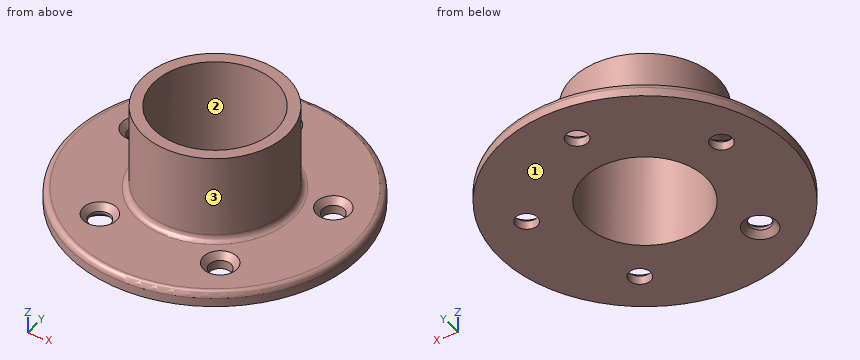
from build123d import *

# Parameters (mm, degrees)
F0_R     = 63.5
F0_R_2   = 4.7625
F0_R_3   = 26.67
F1_DEPTH = 6.35
F2_R     = 31.75
F2_R_2   = 26.67
F3_DEPTH = 38.1
F4_R     = 2.54
F5_SIZE  = 2.54


with BuildPart() as f1:
    # F0 (on Top) → F1 (new body)
    with BuildSketch(Plane.XY):
        Circle(F0_R)
        with Locations((-26.654833, -36.68723)):
            Circle(F0_R_2, mode=Mode.SUBTRACT)
        with Locations((26.654833, -36.68723)):
            Circle(F0_R_2, mode=Mode.SUBTRACT)
        with Locations((-43.128426, 14.013275)):
            Circle(F0_R_2, mode=Mode.SUBTRACT)
        Circle(F0_R_3, mode=Mode.SUBTRACT)
        with Locations((43.128426, 14.013275)):
            Circle(F0_R_2, mode=Mode.SUBTRACT)
        with Locations((0, 45.34791)):
            Circle(F0_R_2, mode=Mode.SUBTRACT)
    extrude(amount=F1_DEPTH)

    # F2 (on face) → F3 (join)
    with BuildSketch(Plane.XY.offset(6.35)):
        Circle(F2_R)
        Circle(F2_R_2, mode=Mode.SUBTRACT)
    extrude(amount=F3_DEPTH)

    # F4
    f4_edges = [f1.edges().sort_by_distance(p)[0] for p in [
        (-31.75, 0, 6.35),
        (-63.5, 0, 6.35),
    ]]
    fillet(f4_edges, radius=F4_R)

    # F5
    f5_edges = [f1.edges().sort_by_distance(p)[0] for p in [
        (-47.890926, 14.013275, 6.35),
        (-21.892333, -36.68723, 3.175),
        (-31.417333, -36.68723, 0),
        (-31.417333, -36.68723, 6.35),
        (21.892333, -36.68723, 6.35),
        (38.365926, 14.013275, 6.35),
        (-4.7625, 45.34791, 6.35),
    ]]
    chamfer(f5_edges, length=F5_SIZE)


solid = f1.part
Read the model definition and answer for the solid it produces. Units are mm, in the model's axes. Face numbers are marked on the shaded views. Round coordinates to 2 decimals unless told otherwise and drop trailing zeros. Order: outer loops, then holes, each group sorted by start corner. A loop starts at its lowest first (then second) coordinate and runs counter-clockwise, first axis right, second up. Notation, with made-up numbers: (-35.5, 48) - (-0.5, 48) arc R26 ccw to (-0.5, 73) - close; hole circle Ø9 at (-35, 55.5). An arc over 180 degrees is marked (long way). Use one line per item in the form item = value. Start each with the question number.
(1) The part is cut by section C-C (z = 39.5). Give the vertices of the cut face in (x, y), then the cut area to 3 significant figures.
(2) Find the intervals of material crossed by line 1 along Y through (x, z) = (0, 1.65); line 2 along Y through (x, z) = (-1, 5.5); line 3 along Y through (x, z) = (0, 31.5), in increasing order. Write a range as from..to.
(3) The part is cut by section A-A (y = 0). Give the vertices of the cut face in (x, z).
(4) Flat-ended cylindrical pins translate along their axes: pin 1 Ø1 at (x, z) = (21.5, 11.5) entering from -Y; pin 2 Ø1 at (y, z) = (5.5, 26.5) entering from +X; pin 3 Ø4 at (y, z) = (16.5, 28) entering from +X. Find the tip coordinate at first contact, or state that the pin passes through.
(5) Determine the mould class of the marked faces 1, 2 and 3 for opening direction Y: +Y half, -Y half, draft (parallel to the pull), parting line (faces both ways), or undercut.
(6) The part is cut by section B-B (x = 0). Give the vertices of the cut face in (y, z), then the cut area to 3 significant figures.
Checked values:
q1.outline = circle Ø63.5 at (0, 0); hole circle Ø53.34 at (0, 0)
q1.area = 932 mm^2
q2.line_1 = -63.5..-26.67, 26.67..40.59, 50.11..63.5
q2.line_2 = -62.85..-26.65, 26.65..38.97, 51.72..62.85
q2.line_3 = -31.75..-26.67, 26.67..31.75
q3.outline = (-63.5, 0) - (-26.67, 0) - (-26.67, 44.45) - (-31.75, 44.45) - (-31.75, 8.89) arc R2.54 cw to (-34.29, 6.35) - (-60.96, 6.35) arc R2.54 ccw to (-63.5, 3.81) - close; (26.67, 0) - (63.5, 0) - (63.5, 3.81) arc R2.54 ccw to (60.96, 6.35) - (34.29, 6.35) arc R2.54 cw to (31.75, 8.89) - (31.75, 44.45) - (26.67, 44.45) - close
q4.pin_1 = -23.81
q4.pin_2 = 31.35
q4.pin_3 = 28.25
q5.face_1 = draft
q5.face_2 = undercut
q5.face_3 = parting line
q6.outline = (-63.5, 0) - (-26.67, 0) - (-26.67, 44.45) - (-31.75, 44.45) - (-31.75, 8.89) arc R2.54 cw to (-34.29, 6.35) - (-60.96, 6.35) arc R2.54 ccw to (-63.5, 3.81) - close; (26.67, 0) - (40.59, 0) - (40.59, 3.81) - (38.05, 6.35) - (34.29, 6.35) arc R2.54 cw to (31.75, 8.89) - (31.75, 44.45) - (26.67, 44.45) - close; (50.11, 0) - (63.5, 0) - (63.5, 3.81) arc R2.54 ccw to (60.96, 6.35) - (52.65, 6.35) - (50.11, 3.81) - close
q6.area = 788 mm^2
